```python
from build123d import *

# Parameters (mm, degrees)
BOSS_EXTRU_1_DEPTH      = 17.9
CONG_1_R                = 9
ENL_V_MAT_EXTRU_1_REACH = 42.145
ENL_V_MAT_EXTRU_2_REACH = 40.414
ESQUISSE3_R             = 1.5
CONG_2_R                = 8


with BuildPart() as part:
    # Esquisse1 → Boss.-Extru.1 (new body)
    with BuildSketch(Plane.XY):
        Polygon((7.5, 4), (30.5, 4), (30.5, -4), (7.5, -4), (7.5, -15), (-7.5, -15), (-7.5, 15), (7.5, 15), align=None)
    extrude(amount=BOSS_EXTRU_1_DEPTH)

    # Congé1
    # the kernel refuses this fillet: 9 mm, written as the material it takes off along each edge
    with BuildSketch(Plane(origin=(30.5, 26.5, 0), x_dir=(0, 0, 1), z_dir=(0, -1, 0))) as cong_1_piece_1:
        with BuildLine():
            CenterArc((CONG_1_R, CONG_1_R), CONG_1_R, 180, 90)
            Line((0, CONG_1_R), (0, 0))
            Line((0, 0), (CONG_1_R, 0))
        make_face()
    extrude(amount=53, mode=Mode.SUBTRACT)
    with BuildSketch(Plane(origin=(30.5, 26.5, 17.9), x_dir=(0, 0, -1), z_dir=(0, -1, 0))) as cong_1_piece_2:
        with BuildLine():
            CenterArc((CONG_1_R, -CONG_1_R), CONG_1_R, 90, 90)
            Line((0, -CONG_1_R), (0, 0))
            Line((0, 0), (CONG_1_R, 0))
        make_face()
    extrude(amount=53, mode=Mode.SUBTRACT)

    # Esquisse2 → Enlèv. mat.-Extru.1 (cut, up to next)
    with BuildSketch(Plane(origin=(0, 4, 0), x_dir=(1, 0, 0), z_dir=(0, 1, 0)), mode=Mode.PRIVATE) as enl_v_mat_extru_1_sk1:
        with BuildLine():
            Line((24.04, -5.84888545), (24.04, -11.95111455))
            ThreePointArc((24.04, -11.95111455), (17.53, -8.9), (24.04, -5.84888545))
        make_face()
    enl_v_mat_extru_1_tool1 = extrude(enl_v_mat_extru_1_sk1.sketch, amount=-ENL_V_MAT_EXTRU_1_REACH, mode=Mode.PRIVATE) & part.part
    add(enl_v_mat_extru_1_tool1.solids().sort_by_distance((21.06418, 4, 8.9))[0], mode=Mode.SUBTRACT)

    # Esquisse3 → Enlèv. mat.-Extru.2 (cut, up to next)
    with BuildSketch(Plane.XY.offset(17.9), mode=Mode.PRIVATE) as enl_v_mat_extru_2_sk1:
        with Locations((0, 10)):
            Circle(ESQUISSE3_R)
    enl_v_mat_extru_2_tool1 = extrude(enl_v_mat_extru_2_sk1.sketch, amount=-ENL_V_MAT_EXTRU_2_REACH, mode=Mode.PRIVATE) & part.part
    # Esquisse3 → Enlèv. mat.-Extru.2 (cut, up to next)
    with BuildSketch(Plane.XY.offset(17.9), mode=Mode.PRIVATE) as enl_v_mat_extru_2_sk2:
        with Locations((0, -10)):
            Circle(ESQUISSE3_R)
    enl_v_mat_extru_2_tool2 = extrude(enl_v_mat_extru_2_sk2.sketch, amount=-ENL_V_MAT_EXTRU_2_REACH, mode=Mode.PRIVATE) & part.part
    add(enl_v_mat_extru_2_tool1.solids().sort_by_distance((0, 10, 17.9))[0], mode=Mode.SUBTRACT)
    add(enl_v_mat_extru_2_tool2.solids().sort_by_distance((0, -10, 17.9))[0], mode=Mode.SUBTRACT)

    # Congé2
    cong_2_edges = [part.edges().sort_by_distance(p)[0] for p in [
        (7.5, 4, 8.95),
        (7.5, -4, 8.95),
    ]]
    fillet(cong_2_edges, radius=CONG_2_R)


solid = part.part
```
Input: part model. Units: mm. Frame: model coordinates. A direction names the side the tool comes from. Give positions to 0.01 mm unless a question says otherwise; leave off trailing zeros. Write each loop counter-clockwise with the first axis right and the second up, starting at its lowest first coordinate (ties: lowest second). Pieces come first, ordered by that corner, then holes. Notation, with made-up numbers: (81, -31) - (135, -31) arc R10 ccw to (135, -14) - close; hole circle Ø9 at (3.5, 80.25). An arc over 180 degrees is marked (long way). Write item = value, one per line. Start each with the question number.
1. Access query for faces 1 (the cylindrical face through (27.776, 0.056, 2.549)), 2 (the flat face through (25, -4, 9)), 3 (the flat face through (24.04, 0, 9)), 4 (the flat face through (7.5, 14, 9)), 5 (the flat face through (4, 0, 17.9)). Directions: +Z, -Z, +X, -X, +Y, -Y. A direction counts if a zero-diameter tool reaches every point of the face in a straight line with its end or side. Return the directions, or none.
2. First-contact query: pin 1 Ø3.5 at (x, y) = (0, 10) entering from -Z; pin 2 Ø3 at (x, z) = (23.5, 8.5) entering from +Y; pin 3 Ø2.5 at (y, z) = (-14, 6.5) entering from +X; pin 4 Ø10 at (x, z) = (26, 7) entering from -Y. Flat tips, straight axial feed; report the tip coordinate or a pass-through.
3. Section query D-D, the plane y = -11. Output: boundary loops of the cut face in (x, z).
4. Section query C-C, the plane x = 0. Output: boundary loops of the cut face in (y, z).
5. Section query B-B, the plane z = 6.5. Output: boundary loops of the cut face in (x, y), then the cut area to 3 significant figures.
6. Ray query, L1, parallel to Y at x = 0, z = 4; L2, parallel to Z at x = 21.5, y = 2.25; L3, parallel to X at y = -12.75, z = 12.75. Return the intervals inside material, ascending.
7. Mould query, pull axis X, two halves, no side actions, for faces 6 (the cylindrical face through (27.92, 0.06, 15.21)), 7 (the cylindrical face through (-0.325, -11.464, 9.075)), 8 (the flat face through (4, 0, 0)), 9 (the cylindrical face through (-0.325, 8.536, 9.075)). Classes: released by +X, released by -X, zero draft, split by the parting line, or undercut.
8. Section query A-A, the plane y = 1.5. Output: boundary loops of the cut face in (x, z).
Check sheet entries:
q1.face_1 = -Z, +X, +Y, -Y
q1.face_2 = +Z, -Z, +X, -Y
q1.face_3 = +Y, -Y
q1.face_4 = +Z, -Z, +X, +Y
q1.face_5 = +Z, +X, -X, +Y, -Y
q2.pin_1 = 0
q2.pin_2 = 4
q2.pin_3 = 7.5
q2.pin_4 = -4
q3.outline = (-7.5, 0) - (-1.12, 0) - (-1.12, 17.9) - (-7.5, 17.9) - close; (1.12, 0) - (7.56, 0) - (7.56, 17.9) - (1.12, 17.9) - close
q4.outline = (-15, 0) - (-11.5, 0) - (-11.5, 17.9) - (-15, 17.9) - close; (-8.5, 0) - (8.5, 0) - (8.5, 17.9) - (-8.5, 17.9) - close; (11.5, 0) - (15, 0) - (15, 17.9) - (11.5, 17.9) - close
q5.outline = (-7.5, -15) - (7.5, -15) - (7.5, -12) arc R8 cw to (15.5, -4) - (18.34, -4) - (18.34, 4) - (15.5, 4) arc R8 cw to (7.5, 12) - (7.5, 15) - (-7.5, 15) - close; (24.04, -4) - (30.15, -4) - (30.15, 4) - (24.04, 4) - close; hole circle Ø3 at (0, -10); hole circle Ø3 at (0, 10)
q5.area = 599 mm2
q6.L1 = -15 to -11.5, -8.5 to 8.5, 11.5 to 15
q6.L2 = 0 to 4.93, 12.87 to 17.9
q6.L3 = -7.5 to 7.5
q7.face_6 = released by +X
q7.face_7 = undercut
q7.face_8 = zero draft
q7.face_9 = undercut
q8.outline = (-7.5, 0) - (21.5, 0) arc R9 ccw to (30.5, 8.95) arc R9 ccw to (21.5, 17.9) - (-7.5, 17.9) - close; hole (24.04, 5.85) - (24.04, 11.95) arc R3.97 ccw (long way) to start
